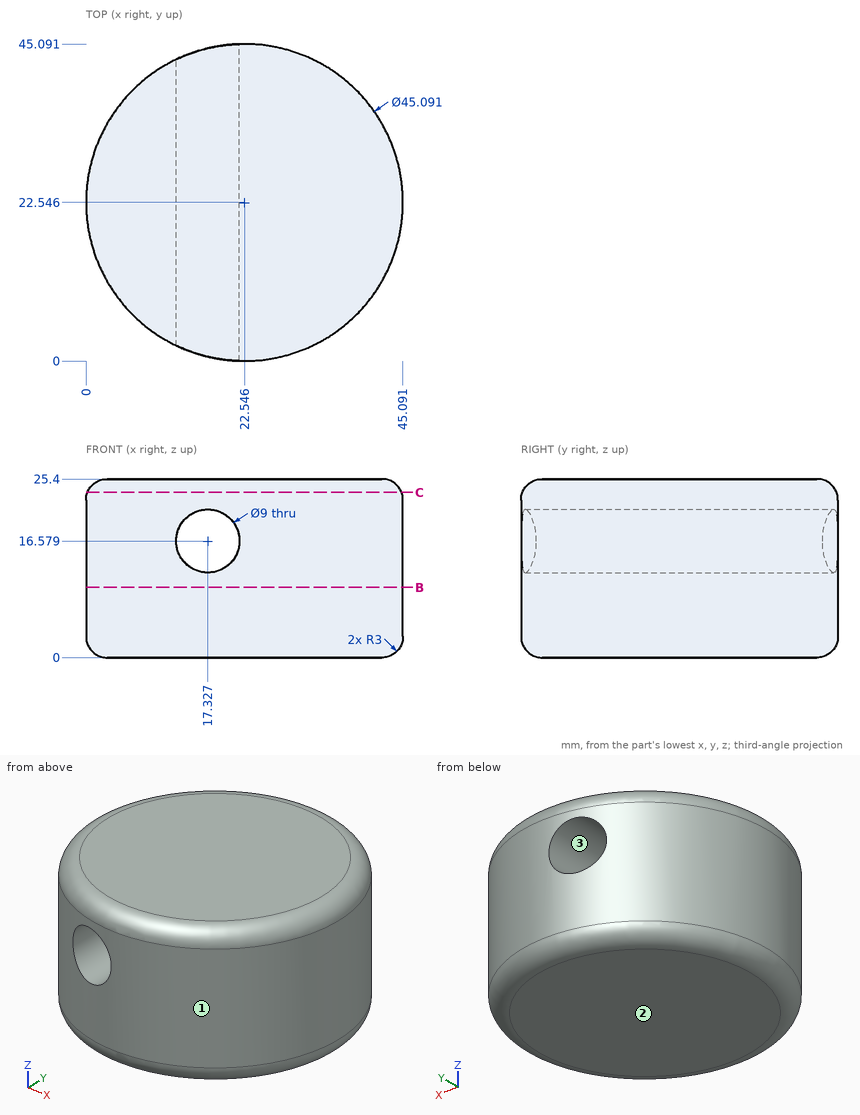
Here's the drawing with two shaded views (mm, measured from the low corner). I have some questions. Coordinates: 2 decimals unless noted, no trailing zeros. Write each loop counter-clockwise with the first axis right and the second up, starting at its lowest first coordinate (ties: lowest second). Pieces come first, ordered by that corner, then holes. Notation, with made-up numbers: (53.25, 51) -> (90.25, 51) arc R18 ccw to (90.25, 73) -> close; hole circle Ø10 at (-39.75, 72). An arc over 180 degrees is marked (long way). One line per question, with ' | ' between items. Start each with the question number.
1. If we section it at B-B (z = 10): Please give me the cut outline in (x, y) (1 decimal), and give its area (3 significant figures).
2. If we section it at C-C (z = 23.5): Please give me the cut outline in (x, y) (1 decimal).
3. Will these pins go through, and if not, where does the flat tip stop? P1, Ø2, axis at x = 14.5, z = 17, coming from the -Y side; P2, Ø2, axis at x = 9, z = 4, coming from the +Y side; P3, Ø6, axis at x = 40, z = 4.5, coming from the -Y side; P4, Ø3, axis at x = 25, z = 21, coming from the +Y side.
4. Please list where these lines run through material, in increasing order: line 1 along X through (y, z) = (34.5, 13.75) (1 decimal); line 2 along X through (y, z) = (23, 18.5) (1 decimal); line 3 along Z through (x, y) = (41.5, 17.5).
5. Thinking about a two-plate mould opening in X: for the marked faces 1, 2 and 3, which applies, pulls with the +X half, pulls with the -X half, needs draft (parallel to the pull), parting line crosses it, or undercut?
Return value:
1) outline: circle Ø45.1 at (22.5, 22.5) | area: 1,600 mm²
2) outline: circle Ø44.7 at (22.5, 22.5)
3) P1: passes through | P2: stops at y = 41.28 | P3: stops at y = 5.24 | P4: stops at y = 45.07
4) line 1: x = 3.4 to 13.8, 20.8 to 41.7 | line 2: x = 0 to 13.3, 21.4 to 45.1 | line 3: z = 0 to 25.4
5) face 1: parting line crosses it | face 2: needs draft | face 3: undercut
